Autodesk Inventor part; units mm, degrees
ref_plane "YZ Plane" through (0, 0, 0) normal (1, 0, 0) x (0, 1, 0)
ref_plane "XZ Plane" through (0, 0, 0) normal (0, 1, 0) x (-1, 0, 0)
ref_plane "XY Plane" through (0, 0, 0) normal (0, 0, 1) x (1, 0, 0)
sketch "スケッチ1" plane through (0, 0, 0) normal (0, 1, 0) x (-1, 0, 0)
  circle A0 centre (0, 0) radius 4
  dimension "d0" = 8
extrude "押し出し1" add sketch "スケッチ1" along normal blind 45
sketch "スケッチ2" plane through (0, 45, 0) normal (0, 1, 0) x (1, 0, 0)
  circle A0 centre (0, 0) radius 1.65
  dimension "d3" = 3.3
extrude "押し出し2" cut sketch "スケッチ2" against normal blind 8
thread "ねじ1"
sketch "スケッチ3" plane through (0, 0, 0) normal (0, -1, 0) x (1, 0, 0)
  circle A0 centre (0, 0) radius 1.65
  dimension "d8" = 3.3
extrude "押し出し3" cut sketch "スケッチ3" against normal blind 8
thread "ねじ2"
fillet "フィレット1" radius 0.3 1 edges at (-1.65, 0, 0)
fillet "フィレット2" radius 0.3 1 edges at (-1.65, 45, 0)
fillet "フィレット3" radius 0.3 2 edges at (4, 45, 0) (4, 0, 0)
properties part number "ARL-445KE"
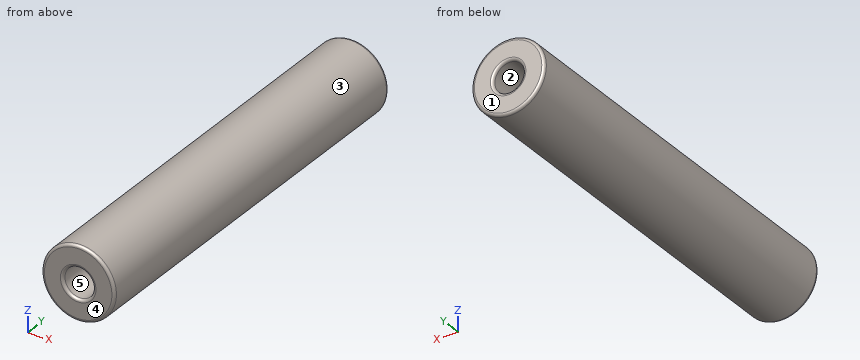
Model file for the job. Use its own axes, mm. Face numbers are marked on the shaded views. A direction names the side the tool comes from. Give positions to 0.01 mm unless a question says otherwise; leave off trailing zeros. Loops run counter-clockwise (first coordinate to the right, second up) from the corner with the lowest first, then second, coordinate; pieces in that order, holes last. Notation, with made-up numbers: M 62.25,-32.5 L 121.25,-32.5 A14 cw 121.25,-26.5 Z; hole C 53.25,86 d4. An arc over 180 degrees is marked long. Use one line per item in the form item = value.
Item 1: Which spindle directions (+Z, -Z, +X, -X, +Y, -Y) get a long thin tool onto all of the face, cutting with end or side? Do the marked faces 4 and 5. Say none if no direction does.
Filled in:
face_4 = +Z, -Z, +X, -X, -Y
face_5 = -Y
Item 2: Drill centre lines: L1, parallel to Z at x = 0, y = 41; L2, parallel to Y at x = -0.5, z = -1.5; L3, parallel to Z at x = 1.5, y = 29. Where is each one in solid material? Low to high.
Filled in:
L1 = -4 to -1.65, 1.65 to 4
L2 = 8 to 37
L3 = -3.71 to 3.71
Item 3: Slice it at B-B on x = 0. List the corners of the cut face in (y, z), and give its area (3 significant figures).
Filled in:
outline = M 0,-3.7 A0.3 ccw 0.3,-4 L 44.7,-4 A0.3 ccw 45,-3.7 L 45,-1.95 A0.3 ccw 44.7,-1.65 L 37,-1.65 L 37,1.65 L 44.7,1.65 A0.3 ccw 45,1.95 L 45,3.7 A0.3 ccw 44.7,4 L 0.3,4 A0.3 ccw 0,3.7 L 0,1.95 A0.3 ccw 0.3,1.65 L 8,1.65 L 8,-1.65 L 0.3,-1.65 A0.3 ccw 0,-1.95 Z
area = 307 mm^2
Item 4: Slice it at A-A on z = 0. List the corners of the cut face in (x, y).
Filled in:
outline = M -4,0.3 A0.3 ccw -3.7,0 L -1.95,0 A0.3 ccw -1.65,0.3 L -1.65,8 L 1.65,8 L 1.65,0.3 A0.3 ccw 1.95,0 L 3.7,0 A0.3 ccw 4,0.3 L 4,44.7 A0.3 ccw 3.7,45 L 1.95,45 A0.3 ccw 1.65,44.7 L 1.65,37 L -1.65,37 L -1.65,44.7 A0.3 ccw -1.95,45 L -3.7,45 A0.3 ccw -4,44.7 Z
Item 5: Flat gauge pins, fed straight in: pin 1 Ø2 at (x, z) = (0, 0) entering from +Y; pin 2 Ø1.5 at (x, y) = (-1.5, 31) entering from +Z. Where does each tip first touch, or does it go through?
Filled in:
pin_1 = 37
pin_2 = 3.93
Item 6: Slice it at D-D on y = 11. List the corners of the cut face in (x, z).
Filled in:
outline = C 0,0 d8
Item 7: Two-plate mould, pull along X, no slides. Class the marked faces 1, 2 and 3: released by +X, released by -X, zero draft, split by the parting line, or undercut.
Filled in:
face_1 = zero draft
face_2 = undercut
face_3 = split by the parting line
Item 8: Slice it at C-C on y = 39.5. List the corners of the cut face in (x, z), and give its area (3 significant figures).
Filled in:
outline = C 0,0 d8; hole C 0,0 d3.3
area = 41.7 mm^2
